Can you work these out from the drawing? Everything is in mm from the part's minimum corner. Give positions to 0.01 mm unless a question says otherwise; leave off trailing zeros. Order: outer loops, then holes, each group sorted by start corner. A loop starts at its lowest first (then second) coordinate and runs counter-clockwise, first axis right, second up. Notation, with made-up numbers: M -27,77.25 L -11,77.25 A31 ccw -11,110.25 Z; hole C 24.25,22.5 d3. An arc over 180 degrees is marked long. Use a Markdown table: item, result. Add a question column.
Item 1: I'm going to push a flat-ended pin straight in: pin 1 Ø1.5 at (y, z) = (3.5, 4.5) entering from -X. Where does the tip first touch, or does it pass through?
Item 2: If I drill on L1, parallel to X at y = 2.1, z = 10; L2, parallel to X at y = 5.1, z = 11.25; L3, parallel to Z at x = 107, y = 1, over which ranges is the centre line in solid material (lowest first)? Write a range as from..to.
Item 3: Suppose I cut it at A-A on x = 107. Write out the boundary of the cut face in (y, z), plus the area to 3 significant figures.
Item 4: Suppose I cut it at B-B on z = 10. Write out the boundary of the cut face in (x, y).
Item 5: Suppose I cut it at C-C on y = 4.55. Write out the boundary of the cut face in (x, z).
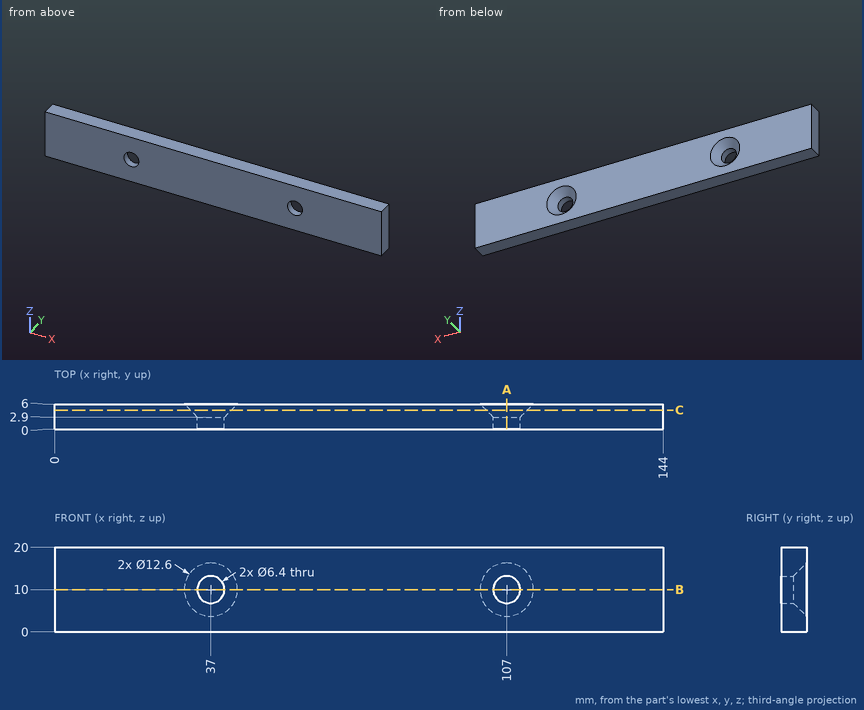
Findings below:
| question | item | result |
|---|---|---|
| 1 | pin 1 | stops at x = 0 |
| 2 | L1 | x = 0..33.8, 40.2..103.8, 110.2..144 |
| 2 | L2 | x = 0..31.75, 42.25..101.75, 112.25..144 |
| 2 | L3 | z = 0..6.8, 13.2..20 |
| 3 | outline | M 0,0 L 6,0 L 6,3.7 L 2.9,6.8 L 0,6.8 Z; M 0,13.2 L 2.9,13.2 L 6,16.3 L 6,20 L 0,20 Z |
| 3 | area | 72.0 mm^2 |
| 4 | outline | M 0,0 L 33.8,0 L 33.8,2.9 L 30.7,6 L 0,6 Z; M 40.2,0 L 103.8,0 L 103.8,2.9 L 100.7,6 L 43.3,6 L 40.2,2.9 Z; M 110.2,0 L 144,0 L 144,6 L 113.3,6 L 110.2,2.9 Z |
| 5 | outline | M 0,0 L 144,0 L 144,20 L 0,20 Z; hole C 37,10 d9.7; hole C 107,10 d9.7 |
